Could you check a few things on this model? Use its own coordinates, in mm. A direction names the side the tool comes from. Coordinates: 2 decimals unless noted, no trailing zeros. Order: outer loops, then holes, each group sorted by start corner. A loop starts at its lowest first (then second) coordinate and runs counter-clockwise, first axis right, second up. Notation, with made-up numbers: (-13, 15.25) - (4, 15.25) arc R26 cw to (4, 51.25) - close; hole circle Ø7 at (30, 4). An arc over 180 degrees is marked (long way). One line per item, written item: value. Start each with the question number.
from build123d import *

# Parameters (mm, degrees)
BOSS_EXTRUDE1_DEPTH = 25
CUT_EXTRUDE1_REACH  = 40.095
SKETCH2_R           = 2
CUT_EXTRUDE2_REACH  = 46.159
SKETCH3_R           = 2


with BuildPart() as part:
    # Sketch1 → Boss-Extrude1 (new body)
    with BuildSketch(Plane.XY):
        with BuildLine():
            Line((0, 0), (35, 0))
            Line((35, 0), (35, 8.5))
            Line((35, 8.5), (23.45, 8.5))
            ThreePointArc((23.45, 8.5), (23.075728652, 10.576956909), (22, 12.392621225))
            Line((22, 12.392621225), (22, 18.5))
            Line((22, 18.5), (18.5, 18.5))
            Line((18.5, 18.5), (18.5, 10.736626925))
            ThreePointArc((18.5, 10.736626925), (17.5, 6.05), (16.5, 10.736626925))
            Line((16.5, 10.736626925), (16.5, 18.5))
            Line((16.5, 18.5), (13, 18.5))
            Line((13, 18.5), (13, 12.392621225))
            ThreePointArc((13, 12.392621225), (11.924271348, 10.576956909), (11.55, 8.5))
            Line((11.55, 8.5), (0, 8.5))
            Line((0, 8.5), (0, 0))
        make_face()
    extrude(amount=BOSS_EXTRUDE1_DEPTH)

    # Cut-Extrude1: up to this face of the body (flat: up to its plane)
    cut_extrude1_end = Plane(part.part.faces().sort_by_distance((13, 15.446310612, 12.5))[0])
    # Sketch2 → Cut-Extrude1 (cut, up to the picked face)
    with BuildSketch(Plane(origin=(22, 0, 0), x_dir=(0, 0, -1), z_dir=(1, 0, 0)), mode=Mode.PRIVATE) as cut_extrude1_sk1:
        with Locations(Location((-18, 15.446310612, 0), (0, 0, 90))):
            Circle(SKETCH2_R)
    cut_extrude1_tool1 = split(extrude(cut_extrude1_sk1.sketch, amount=-CUT_EXTRUDE1_REACH, mode=Mode.PRIVATE), bisect_by=cut_extrude1_end, keep=Keep.BOTH, mode=Mode.PRIVATE)
    # Sketch2 → Cut-Extrude1 (cut, up to the picked face)
    with BuildSketch(Plane(origin=(22, 0, 0), x_dir=(0, 0, -1), z_dir=(1, 0, 0)), mode=Mode.PRIVATE) as cut_extrude1_sk2:
        with Locations(Location((-7, 15.446310612, 0), (0, 0, 90))):
            Circle(SKETCH2_R)
    cut_extrude1_tool2 = split(extrude(cut_extrude1_sk2.sketch, amount=-CUT_EXTRUDE1_REACH, mode=Mode.PRIVATE), bisect_by=cut_extrude1_end, keep=Keep.BOTH, mode=Mode.PRIVATE)
    add(cut_extrude1_tool1.solids().sort_by(Axis((22, 15.446311, 18), (-1, 0, 0)))[0], mode=Mode.SUBTRACT)
    add(cut_extrude1_tool2.solids().sort_by(Axis((22, 15.446311, 7), (-1, 0, 0)))[0], mode=Mode.SUBTRACT)

    # Sketch3 → Cut-Extrude2 (cut, up to next)
    with BuildSketch(Plane(origin=(0, 8.5, 0), x_dir=(1, 0, 0), z_dir=(0, 1, 0)), mode=Mode.PRIVATE) as cut_extrude2_sk1:
        with Locations(Location((29.225, -18, 0), (0, 0, 180))):
            Circle(SKETCH3_R)
    cut_extrude2_tool1 = extrude(cut_extrude2_sk1.sketch, amount=-CUT_EXTRUDE2_REACH, mode=Mode.PRIVATE) & part.part
    # Sketch3 → Cut-Extrude2 (cut, up to next)
    with BuildSketch(Plane(origin=(0, 8.5, 0), x_dir=(1, 0, 0), z_dir=(0, 1, 0)), mode=Mode.PRIVATE) as cut_extrude2_sk2:
        with Locations(Location((29.225, -7, 0), (0, 0, 180))):
            Circle(SKETCH3_R)
    cut_extrude2_tool2 = extrude(cut_extrude2_sk2.sketch, amount=-CUT_EXTRUDE2_REACH, mode=Mode.PRIVATE) & part.part
    # Sketch3 → Cut-Extrude2 (cut, up to next)
    with BuildSketch(Plane(origin=(0, 8.5, 0), x_dir=(1, 0, 0), z_dir=(0, 1, 0)), mode=Mode.PRIVATE) as cut_extrude2_sk3:
        with Locations(Location((5.775, -7, 0), (0, 0, 270))):
            Circle(SKETCH3_R)
    cut_extrude2_tool3 = extrude(cut_extrude2_sk3.sketch, amount=-CUT_EXTRUDE2_REACH, mode=Mode.PRIVATE) & part.part
    # Sketch3 → Cut-Extrude2 (cut, up to next)
    with BuildSketch(Plane(origin=(0, 8.5, 0), x_dir=(1, 0, 0), z_dir=(0, 1, 0)), mode=Mode.PRIVATE) as cut_extrude2_sk4:
        with Locations(Location((5.775, -18, 0), (0, 0, 270))):
            Circle(SKETCH3_R)
    cut_extrude2_tool4 = extrude(cut_extrude2_sk4.sketch, amount=-CUT_EXTRUDE2_REACH, mode=Mode.PRIVATE) & part.part
    add(cut_extrude2_tool1.solids().sort_by_distance((29.225, 8.5, 18))[0], mode=Mode.SUBTRACT)
    add(cut_extrude2_tool2.solids().sort_by_distance((29.225, 8.5, 7))[0], mode=Mode.SUBTRACT)
    add(cut_extrude2_tool3.solids().sort_by_distance((5.775, 8.5, 7))[0], mode=Mode.SUBTRACT)
    add(cut_extrude2_tool4.solids().sort_by_distance((5.775, 8.5, 18))[0], mode=Mode.SUBTRACT)


solid = part.part
Q1. Which directions (+Z, -Z, +X, -X, +Y, -Y) give clear straight access to the entire face, cutting with the end or side of a thin tool? Please do faces 1 (the flat face through (16.5, 15, 12)), 2 (the flat face through (6, 8.5, 12)), 3 (the flat face through (22, 15, 12)).
Q2. I want a section at D-D on y = 9.75. Please give me the cut outline in (x, z), then the cut area to 3 significant figures.
Q3. I want a section at C-C on x = 30. Please give me the cut outline in (y, z), then the cut area to 3 significant figures.
Q4. I want a section at A-A on z = 7. State how many separate pieces and enclosed holes the cut face has, then the cut area to 3 significant figures.
Q5. If I drill on L1, parallel to Z at x = 30.5, y = 1; L2, parallel to X at y = 17.75, z = 15.5; L3, parallel to Z at x = 4, y = 7, over which ranges is the centre line in solid material (lowest first)?
Q6. I want a section at B-B on y = 14.5. Please give me the cut outline in (x, z).
Q7. We'd pull the mould along Z, two halves only. Please class faces 4 (the flat face through (0, 4, 12)), 5 (the cylindrical face through (20.274, 17.354, 7.601)), 6 (the flat face through (17, 5, 25)): +Z half, -Z half, draft (parallel to the pull), parting line (faces both ways), or undercut.
Q8. I'm going to push flat-ended pins straight in: pin 1 (1.8 mm diameter, centred on y = 14.5, z = 11.5, fed in from +X); pin 2 (5 mm diameter, centred on x = 16.5, y = 13.5, fed in from -Z); pin 3 (12 mm diameter, centred on x = 5.5, z = 17.5, fed in from +Y); pin 4 (2.5 mm diameter, centred on y = 14, z = 14.5, fed in from -X). Where does each tip first touch, or does it pass through?
Values follow:
1. face 1: +Z, -Z, +Y
1. face 2: +Z, -Z, -X, +Y
1. face 3: +Z, -Z, +X, +Y
2. outline: (11.68, 0) - (15.39, 0) - (15.39, 25) - (11.68, 25) - close; (19.61, 0) - (23.32, 0) - (23.32, 25) - (19.61, 25) - close
2. area: 186 mm^2
3. outline: (0, 0) - (8.5, 0) - (8.5, 5.16) - (0, 5.16) - close; (0, 8.84) - (8.5, 8.84) - (8.5, 16.16) - (0, 16.16) - close; (0, 19.84) - (8.5, 19.84) - (8.5, 25) - (0, 25) - close
3. area: 150 mm^2
4. separate pieces: 5
4. enclosed holes: 0
4. area: 265 mm^2
5. L1: z = 0 to 5.46, 8.54 to 16.46, 19.54 to 25
5. L2: x = 13 to 16.5, 18.5 to 22
5. L3: z = 0 to 6.08, 7.92 to 17.08, 18.92 to 25
6. outline: (13, 0) - (16.5, 0) - (16.5, 5.24) - (13, 5.24) - close; (13, 8.76) - (16.5, 8.76) - (16.5, 16.24) - (13, 16.24) - close; (13, 19.76) - (16.5, 19.76) - (16.5, 25) - (13, 25) - close; (18.5, 0) - (22, 0) - (22, 5.24) - (18.5, 5.24) - close; (18.5, 8.76) - (22, 8.76) - (22, 16.24) - (18.5, 16.24) - close; (18.5, 19.76) - (22, 19.76) - (22, 25) - (18.5, 25) - close
7. face 4: draft
7. face 5: undercut
7. face 6: +Z half
8. pin 1: stops at x = 22
8. pin 2: stops at z = 0
8. pin 3: stops at y = 8.5
8. pin 4: stops at x = 13
